Check sheet for the modelled part. Datum: model origin and axes. Units: mm. A direction names the side the tool comes from. Give positions to 0.01 mm unless a question says otherwise; leave off trailing zeros. Order: outer loops, then holes, each group sorted by start corner. A loop starts at its lowest first (then second) coordinate and runs counter-clockwise, first axis right, second up. Notation, with made-up numbers: (2, 14) -> (43, 14) arc R19 cw to (43, 43) -> close; hole circle Ø10 at (80.5, 56.25). An arc over 180 degrees is marked (long way). One line per question, with ' | ' between items.
```python
from build123d import *

# Parameters (mm, degrees)
CHANFREIN1_SIZE = 0.5
CONG_1_R        = 1


with BuildPart() as part:
    # Esquisse1 → Révolution1 (revolve)
    with BuildSketch(Plane.XY):
        with BuildLine():
            Line((-5.830951895, -18.5), (-10, -18.5))
            Line((-10, -18.5), (-10, -2.5))
            Line((-10, -2.5), (-3, -2.5))
            Line((-3, -2.5), (-3, 22.5))
            Line((-3, 22.5), (0, 22.5))
            Line((0, 22.5), (0, -22.5))
            ThreePointArc((0, -22.5), (-3.535533906, -21.403882032), (-5.830951895, -18.5))
        make_face()
    revolve(axis=Axis((0, 22.5, 0), (0, -1, 0)))

    # Chanfrein1
    chanfrein1_edges = [part.edges().sort_by_distance(p)[0] for p in [
        (3, 22.5, 0),
    ]]
    chamfer(chanfrein1_edges, length=CHANFREIN1_SIZE)

    # Congé1
    cong_1_edges = [part.edges().sort_by_distance(p)[0] for p in [
        (10, -18.5, 0),
    ]]
    fillet(cong_1_edges, radius=CONG_1_R)


solid = part.part
```
Q1. Section check A-A (x = 0). Enter the section's corners in (y, z).
Result sheet:
outline: (-18.5, -9) arc R1 ccw to (-17.5, -10) -> (-2.5, -10) -> (-2.5, -3) -> (22, -3) -> (22.5, -2.5) -> (22.5, 2.5) -> (22, 3) -> (-2.5, 3) -> (-2.5, 10) -> (-17.5, 10) arc R1 ccw to (-18.5, 9) -> (-18.5, 5.83) arc R6.25 ccw to (-18.5, -5.83) -> close
Q2. Section check C-C (y = -3.5). Enter the section's corners in (x, z), and give its area (3 significant figures).
Result sheet:
outline: circle Ø20 at (0, 0) | area: 314 mm2
Q3. Thickness scan on line 1 (Y direction, x = 6.5, z = 3); line 2 (X direction, y = -0.5, z = 2.75); line 3 (X direction, y = 17.5, z = 2.25). Record the ranges inside material, lowest first.
Result sheet:
line 1: y = -18.5 to -2.5 | line 2: x = -1.2 to 1.2 | line 3: x = -1.98 to 1.98
Q4. Access from +Z, -Z, +X, -X, +Y, -Y to the whole of each face (thin tool, end or side, straight path). Record for faces 1 (the face through (0, 22.5, 0)), 2 (the face through (3, 10, 0)), 3 (the face through (0, -18.5, 6)).
Result sheet:
face 1: +Z, -Z, +X, -X, +Y | face 2: +Y | face 3: -Y
Q5. Section check B-B (z = 0). Enter the section's corners in (x, y).
Result sheet:
outline: (-10, -17.5) arc R1 ccw to (-9, -18.5) -> (-5.83, -18.5) arc R6.25 ccw to (5.83, -18.5) -> (9, -18.5) arc R1 ccw to (10, -17.5) -> (10, -2.5) -> (3, -2.5) -> (3, 22) -> (2.5, 22.5) -> (-2.5, 22.5) -> (-3, 22) -> (-3, -2.5) -> (-10, -2.5) -> close
Q6. Section check D-D (y = 5.5). Enter the section's corners in (x, z).
Result sheet:
outline: circle Ø6 at (0, 0)
Q7. Depth check by flat-ended pin: pin 1 Ø2 at (x, z) = (6, 2) entering from +Y; pin 2 Ø1 at (x, z) = (6, 0) entering from -Y; pin 3 Ø4 at (x, z) = (8, -7) entering from -Y; pin 4 Ø6 at (y, z) = (-17.5, 0.5) entering from -X. Enter the tip coordinate at first touch or a pass-through.
Result sheet:
pin 1: stops at y = -2.5 | pin 2: stops at y = -19.22 | pin 3: stops at y = -18.5 | pin 4: stops at x = -10
